Check sheet for the modelled part. Datum: model origin and axes. Units: mm. A direction names the side the tool comes from. Round coordinates to 2 decimals unless told otherwise and drop trailing zeros. Loops run counter-clockwise (first coordinate to the right, second up) from the corner with the lowest first, then second, coordinate; pieces in that order, holes last. Notation, with made-up numbers: (-37, 0) - (2, 0) arc R15 ccw to (2, 6) - close; hole circle Ø7 at (44, 24.5). An arc over 180 degrees is marked (long way). Return JSON: item names as keys, results as strings.
from build123d import *

# Parameters (mm, degrees)
EXTRUDE_2_DEPTH = 1.8
EXTRUDE_3_DEPTH = 6


with BuildPart() as part:
    # 草图3 → 凸台-拉伸2 (new body)
    with BuildSketch(Plane(origin=(0, 0, 0), x_dir=(1, 0, 0), z_dir=(0, 1, 0))):
        with BuildLine():
            Line((-12.727922061, 4.5), (-4.5, 4.5))
            Line((-4.5, 4.5), (-4.5, 12.727922061))
            ThreePointArc((-4.5, 12.727922061), (0, 13.5), (4.5, 12.727922061))
            Line((4.5, 12.727922061), (4.5, 4.5))
            Line((4.5, 4.5), (12.703836594, 4.567552496))
            ThreePointArc((12.703836594, 4.567552496), (13.499952375, 0.035858923), (12.727922061, -4.5))
            Line((12.727922061, -4.5), (4.5, -4.5))
            Line((4.5, -4.5), (4.5, -12.741400862))
            ThreePointArc((4.5, -12.741400862), (0, -13.512708682), (-4.5, -12.741400862))
            Line((-4.5, -12.741400862), (-4.5, -4.5))
            Line((-4.5, -4.5), (-12.727922061, -4.5))
            ThreePointArc((-12.727922061, -4.5), (-13.5, 0), (-12.727922061, 4.5))
        make_face()
    extrude(amount=EXTRUDE_2_DEPTH)

    # 草图4 → 凸台-拉伸3 (add)
    with BuildSketch(Plane(origin=(0, 1.8, 0), x_dir=(1, 0, 0), z_dir=(0, 1, 0))):
        Polygon((3.9, -11.7), (-3.9, -11.7), (-3.9, -3.9), (-11.7, -3.9), (-11.7, 3.9), (-3.9, 3.9), (-3.9, 11.7), (3.9, 11.7), (3.9, 3.9), (11.7, 3.9), (11.7, -3.9), (3.9, -3.9), align=None)
    extrude(amount=EXTRUDE_3_DEPTH)


solid = part.part
Q1. Sectioned sample at B-B (z = -8.5). Enter the section's corners in (x, y).
Answer key:
{"outline": "(-4.5, 0) - (4.5, 0) - (4.5, 1.8) - (3.9, 1.8) - (3.9, 7.8) - (-3.9, 7.8) - (-3.9, 1.8) - (-4.5, 1.8) - close"}
Q2. Depth check by flat-ended pin: P1, Ø1.4, axis at y = 1, z = -10.5, coming from the -X side; P2, Ø3, axis at y = 4.5, z = 7.5, coming from the +X side; P3, Ø1, axis at x = -7, y = 4, coming from the +Z side. Enter the tip coordinate at first touch or a pass-through.
Answer key:
{"P1": "stops at x = -4.5", "P2": "stops at x = 3.9", "P3": "stops at z = 3.9"}
Q3. Sectioned sample at A-A (y = 5.5). Enter the section's corners in (x, z).
Answer key:
{"outline": "(-11.7, -3.9) - (-3.9, -3.9) - (-3.9, -11.7) - (3.9, -11.7) - (3.9, -3.9) - (11.7, -3.9) - (11.7, 3.9) - (3.9, 3.9) - (3.9, 11.7) - (-3.9, 11.7) - (-3.9, 3.9) - (-11.7, 3.9) - close"}
Q4. Sectioned sample at C-C (x = -3). Enter the section's corners in (y, z), plus the area to 3 significant figures.
Answer key:
{"outline": "(0, -13.16) - (1.8, -13.16) - (1.8, -11.7) - (7.8, -11.7) - (7.8, 11.7) - (1.8, 11.7) - (1.8, 13.18) - (0, 13.18) - close", "area": "188 mm²"}
Q5. Scan lines: probe 1 along X at (y, z) = (4, -2.25); probe 2 along X at (y, z) = (5, 8.25). Record each from-to range of solid material in increasing order. Write a range as [from, to].
Answer key:
{"probe 1": "x = [-11.7, 11.7]", "probe 2": "x = [-3.9, 3.9]"}
Q6. Tool access check on faces 1 (the face through (8, 5, -3.9)), 2 (the face through (3.9, 5, 8)), 3 (the face through (-4.5, 1, 9)), 4 (the face through (-3.9, 5, -8)). Record the directions out of +Z, -Z, +X, -X, +Y, -Y that give a thin tool (end or side, any length) a straight path to the whole face; none if there is none.
Answer key:
{"face 1": "-Z, +X, +Y", "face 2": "+Z, +X, +Y", "face 3": "+Z, -X, +Y, -Y", "face 4": "-Z, -X, +Y"}
